For this review, take the finished solid that the model builds, in its own axes (mm). Face numbers are marked on the shaded views. A direction names the side the tool comes from. Give positions to 0.01 mm unless a question says otherwise; leave off trailing zeros. Order: outer loops, then holes, each group sorted by start corner. A loop starts at its lowest first (then second) coordinate and runs counter-clockwise, first axis right, second up. Notation, with made-up numbers: M 85.25,-30 L 125.25,-30 A31 cw 125.25,-2 Z; hole C 17,-23 d9. An arc over 180 degrees is marked long. Answer as CSV lines item,"result". Start each with the question number.
1. We need section C-C, the plane z = -239.5. Give the boundary of the cut face in (x, y), and give its area (3 significant figures).
2. Mouldability with a two-part tool opening along Z and no side actions: class the marked faces 4, 5 and 6 as pulls with the +Z half, pulls with the -Z half, needs draft (parallel to the pull), parting line crosses it, or undercut.
3. Machinability: for the marked faces 1, 2 and 3, which of the approach directions +Z, -Z, +X, -X, +Y, -Y give a long, thin tool a straight path to every point of the face, cutting with its end or side? Answer none if there is none.
4. We need section B-B, the plane x = 112. Give the boundary of the cut face in (y, z), and give its area (3 significant figures).
5. For line 1 along Z through (x, y) = (-180.5, -360.5); line 2 along Z through (x, y) = (-129, 109.5), list the stretches that pass through material, from the lowest coordinate up.
6. Clearance check with flat-ended pins moving along their axes: P1, Ø5, axis at y = 209.5, z = 72, coming from the +X side; P2, Ø4, axis at x = -181.5, y = -110.5, coming from the +Z side; P3, Ø12, axis at y = 173.5, z = 42.5, coming from the +X side. State where each tip first meets the part, or that it passes through.
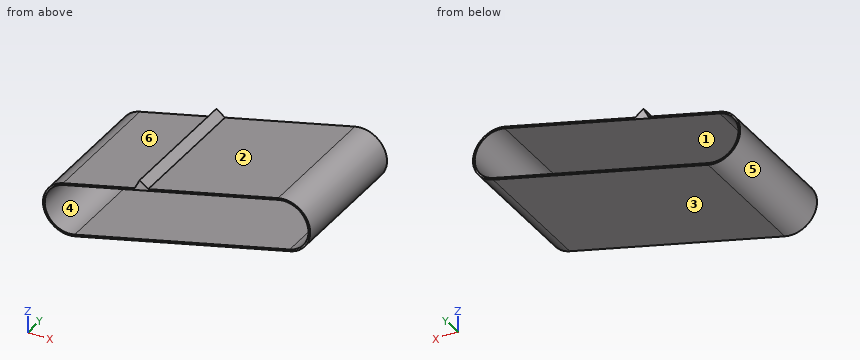
from build123d import *

# Parameters (mm, degrees)
PAD_DEPTH = 800


with BuildPart() as part:
    # Sketch → Pad (new body)
    with BuildSketch(Plane.XZ.offset(400)):
        with BuildLine():
            Line((-670.82039, 0), (-247.213593, 100))
            Line((-247.213593, 100), (-218.661794, 156.72588))
            Line((-218.661794, 156.72588), (-167.755704, 118.757463))
            Line((-167.755704, 118.757463), (600, 300))
            ThreePointArc((670.820393, 1e-06), (785.410194, 185.410196), (600, 300))
            Line((-600, -300), (670.820393, 1e-06))
            ThreePointArc((-670.82039, 0), (-785.410196, -185.410195), (-600, -300))
        make_face()
        with BuildLine():
            Line((-668.459715, -10), (602.360681, 290.000001))
            ThreePointArc((668.4598, 10.00002), (775.410185, 183.04956), (602.360681, 290.000001))
            Line((-602.360681, -290.000002), (668.4598, 10.00002))
            ThreePointArc((-668.459715, -10), (-775.410197, -183.049518), (-602.360681, -290.000002))
        make_face(mode=Mode.SUBTRACT)
    extrude(amount=-PAD_DEPTH)


solid = part.part
Result set:
1,outline,"M -760.88,-400 L -748.02,-400 L -748.02,400 L -760.88,400 Z; M -388.44,-400 L -343.72,-400 L -343.72,400 L -388.44,400 Z"
1,area,"46,100 mm2"
2,face 4,"undercut"
2,face 5,"parting line crosses it"
2,face 6,"pulls with the +Z half"
3,face 1,"+Y, -Y"
3,face 2,"+Z, +Y, -Y"
3,face 3,"-Z, +X, +Y, -Y"
4,outline,"M -400,-131.92 L 400,-131.92 L 400,-121.36 L -400,-121.36 Z; M -400,174.24 L 400,174.24 L 400,184.8 L -400,184.8 Z"
4,area,"16,900 mm2"
5,line 1,"-200.97 to -190.41, 105.19 to 128.26"
5,line 2,"-188.81 to -178.25, 117.35 to 127.91"
6,P1,"x = 769.77"
6,P2,"z = 130.5"
6,P3,"x = 751.39"
